```python
from build123d import *

# Parameters (mm, degrees)
F0_R     = 4.765
F1_DEPTH = 4


with BuildPart() as f1:
    # F0 (on Front) → F1 (new body)
    with BuildSketch(Plane.XZ):
        with BuildLine():
            ThreePointArc((-0.13718, 14.035607), (-10.720514, 12.106821), (-21.303847, 14.035607))
            ThreePointArc((-21.303847, 14.035607), (-41.595514, 0), (-21.303847, -14.035607))
            ThreePointArc((-21.303847, -14.035607), (-10.720514, -12.106821), (-0.13718, -14.035607))
            ThreePointArc((-0.13718, -14.035607), (20.154486, 0), (-0.13718, 14.035607))
        make_face()
        with Locations((-26.595514, 0)):
            Circle(F0_R, mode=Mode.SUBTRACT)
        with BuildLine():
            ThreePointArc((9.919486, 0), (5.154486, -4.765), (0.389486, 0))
            ThreePointArc((0.389486, 0), (5.154486, 4.765), (9.919486, 0))
        make_face(mode=Mode.SUBTRACT)
    extrude(amount=-F1_DEPTH)


solid = f1.part
```
Read the model definition and answer for the solid it produces. Units are mm, in the model's axes. Give positions to 0.01 mm unless a question says otherwise; leave off trailing zeros. Write each loop counter-clockwise with the first axis right and the second up, starting at its lowest first coordinate (ties: lowest second). Pieces come first, ordered by that corner, then holes. Notation, with made-up numbers: M 68,-8 L 117,-8 A18 ccw 117,11 Z; hole C -8.5,-10 d6. An arc over 180 degrees is marked long. Put each result on its own line as item: value. Start each with the question number.
1. The part is cut by section A-A, the plane z = 0. Give the vertices of the cut face in (x, y), and give its area (3 significant figures).
2. Consider line 1 along Z through (x, y) = (-27.5, 1.75); line 2 along Z through (x, y) = (-30.5, 1.55); line 3 along Z through (x, y) = (-35.5, 1.8). Determine where each line is inside the solid, lowest interval first.
3. For a pull along X with two mould halves and no side action, classify faces 1 (the flat face through (-11, 4, 0)), 2 (the cylindrical face through (-22.05, 1.97, 1.43)) as released by +X, released by -X, zero draft, split by the parting line, or undercut.
4. The part is cut by section D-D, the plane z = -4. Give the vertices of the cut face in (x, y).
5. The part is cut by section B-B, the plane x = 8. Give the vertices of the cut face in (y, z), and give its area (3 significant figures).
6. The part is cut by section C-C, the plane y = 2.15. Give the vertices of the cut face in (x, z) (3 decimals).
Final values:
1. outline: M -41.6,0 L -31.36,0 L -31.36,4 L -41.6,4 Z; M -21.83,0 L 0.39,0 L 0.39,4 L -21.83,4 Z; M 9.92,0 L 20.15,0 L 20.15,4 L 9.92,4 Z
1. area: 171 mm²
2. line 1: z = -14.97 to -4.68, 4.68 to 14.97
2. line 2: z = -14.48 to -2.73, 2.73 to 14.48
2. line 3: z = -12.07 to 12.07
3. face 1: zero draft
3. face 2: undercut
4. outline: M -41.05,0 L -29.18,0 L -29.18,4 L -41.05,4 Z; M -24.01,0 L 2.57,0 L 2.57,4 L -24.01,4 Z; M 7.74,0 L 19.61,0 L 19.61,4 L 7.74,4 Z
5. outline: M 0,-14.73 L 4,-14.73 L 4,-3.82 L 0,-3.82 Z; M 0,3.82 L 4,3.82 L 4,14.73 L 0,14.73 Z
5. area: 87.2 mm²
6. outline: M -21.304,-14.036 A30 cw -0.137,-14.036 A15 ccw long -0.137,14.036 A30 cw -21.304,14.036 A15 ccw long Z; hole C -26.596,0 d9.53; hole C 5.154,0 d9.53
